from build123d import *

# Parameters (mm, degrees)
SKETCH_1_W         = 31
SKETCH_1_H         = 21
EXTRUDE_1_DEPTH    = 42
SHELL_1_T          = -1
SKETCH_2_W         = 5
SKETCH_2_H         = 21
EXTRUDE_2_DEPTH    = 6
SHELL_START        = 42
SHELL_2_OUTLINE_W  = 4
SHELL_2_OUTLINE_H  = 21
SHELL_2_DEPTH      = 6
SKETCH_3_W         = 5
SKETCH_3_H         = 21
EXTRUDE_3_DEPTH    = 6
SHELL_START_2      = -6
SHELL_3_OUTLINE_W  = 4
SHELL_3_OUTLINE_H  = 21
SHELL_3_DEPTH      = 6
SKETCH_4_W         = 21
SKETCH_4_H         = 1
EXTRUDE_4_DEPTH    = 23
SKETCH_5_W         = 21
SKETCH_5_H         = 5
EXTRUDE_5_DEPTH    = 6
SHELL_START_3      = 18
SHELL_4_OUTLINE_W  = 21
SHELL_4_OUTLINE_H  = 6
SHELL_4_DEPTH      = 4
SKETCH_6_W         = 21
SKETCH_6_H         = 5
EXTRUDE_6_DEPTH    = 6
SHELL_5_OUTLINE_W  = 21
SHELL_5_OUTLINE_H  = 6
SHELL_5_DEPTH      = 4
SKETCH_8_W         = 21
SKETCH_8_H         = 42
EXTRUDE_7_DEPTH    = 1
HOLE_WIZARD_M3_1_D = 2.5
HOLE_WIZARD_M3_2_D = 2.5
HOLE_WIZARD_M3_3_D = 2.5
HOLE_WIZARD_M3_4_D = 2.5
FILLET_2_R         = 0.5
FILLET_3_R         = 5


# Read off the part's stored shape, not the designer's step: 抽壳2, 抽壳3, 抽壳4, 抽壳5
with BuildPart() as part:
    # 草图1 → 凸台-拉伸1 (new body)
    with BuildSketch(Plane(origin=(0, 0, 0), x_dir=(1, 0, 0), z_dir=(0, 1, 0))):
        with Locations((-15.5, 10.5)):
            Rectangle(SKETCH_1_W, SKETCH_1_H)
    extrude(amount=EXTRUDE_1_DEPTH)

    # 抽壳1
    shell_1_openings = [part.faces().sort_by_distance(p)[0] for p in [
        (-15.5, 21, 0),
        (-31, 21, -10.5),
        (-15.5, 21, -21),
    ]]
    offset(amount=SHELL_1_T, openings=shell_1_openings, kind=Kind.INTERSECTION)

    # 草图2 → 凸台-拉伸2 (add)
    with BuildSketch(Plane(origin=(0, 42, 0), x_dir=(1, 0, 0), z_dir=(0, 1, 0))):
        with Locations((-28.5, 10.5)):
            Rectangle(SKETCH_2_W, SKETCH_2_H)
    extrude(amount=EXTRUDE_2_DEPTH)

    # 抽壳2 outline → 抽壳2 (cut)
    with BuildSketch(Plane(origin=(0, 0, 0), x_dir=(1, 0, 0), z_dir=(0, 1, 0)).offset(SHELL_START)):
        with Locations((-28, 10.5)):
            Rectangle(SHELL_2_OUTLINE_W, SHELL_2_OUTLINE_H)
    extrude(amount=SHELL_2_DEPTH, mode=Mode.SUBTRACT)

    # 草图3 → 凸台-拉伸3 (add)
    with BuildSketch(Plane.XZ):
        with Locations((-28.5, -10.5)):
            Rectangle(SKETCH_3_W, SKETCH_3_H)
    extrude(amount=EXTRUDE_3_DEPTH)

    # 抽壳3 outline → 抽壳3 (cut)
    with BuildSketch(Plane(origin=(0, 0, 0), x_dir=(1, 0, 0), z_dir=(0, 1, 0)).offset(SHELL_START_2)):
        with Locations((-28, 10.5)):
            Rectangle(SHELL_3_OUTLINE_W, SHELL_3_OUTLINE_H)
    extrude(amount=SHELL_3_DEPTH, mode=Mode.SUBTRACT)

    # 草图4 → 凸台-拉伸4 (add)
    with BuildSketch(Plane.XY):
        with Locations((-19.5, 41.5)):
            Rectangle(SKETCH_4_W, SKETCH_4_H)
        with Locations((-19.5, 0.5)):
            Rectangle(SKETCH_4_W, SKETCH_4_H)
    extrude(amount=EXTRUDE_4_DEPTH)

    # 草图5 → 凸台-拉伸5 (add)
    with BuildSketch(Plane(origin=(0, 42, 0), x_dir=(1, 0, 0), z_dir=(0, 1, 0))):
        with Locations((-19.5, -20.5)):
            Rectangle(SKETCH_5_W, SKETCH_5_H)
    extrude(amount=EXTRUDE_5_DEPTH)

    # 抽壳4 outline → 抽壳4 (cut)
    with BuildSketch(Plane.XY.offset(SHELL_START_3)):
        with Locations((-19.5, 45)):
            Rectangle(SHELL_4_OUTLINE_W, SHELL_4_OUTLINE_H)
    extrude(amount=SHELL_4_DEPTH, mode=Mode.SUBTRACT)

    # 草图6 → 凸台-拉伸6 (add)
    with BuildSketch(Plane.XZ):
        with Locations((-19.5, 20.5)):
            Rectangle(SKETCH_6_W, SKETCH_6_H)
    extrude(amount=EXTRUDE_6_DEPTH)

    # 抽壳5 outline → 抽壳5 (cut)
    with BuildSketch(Plane.XY.offset(SHELL_START_3)):
        with Locations((-19.5, -3)):
            Rectangle(SHELL_5_OUTLINE_W, SHELL_5_OUTLINE_H)
    extrude(amount=SHELL_5_DEPTH, mode=Mode.SUBTRACT)

    # 草图8 → 凸台-拉伸7 (add)
    with BuildSketch(Plane(origin=(0, 0, -21), x_dir=(-1, 0, 0), z_dir=(0, 0, -1))):
        with Locations((19.5, 21)):
            Rectangle(SKETCH_8_W, SKETCH_8_H)
    extrude(amount=EXTRUDE_7_DEPTH)

    # M3 螺纹孔1 (through all)
    with Locations(Plane.XY.offset(23)):
        with Locations((-24.5, 45), (-14.5, 45), (-24.5, -3), (-14.5, -3)):
            Hole(HOLE_WIZARD_M3_1_D / 2)

    # M3 螺纹孔2 (through all)
    with Locations(Plane.ZY.offset(31)):
        with Locations((-5.5, 45), (-15.5, 45), (-15.5, -3), (-5.5, -3)):
            Hole(HOLE_WIZARD_M3_2_D / 2)

    # M3 螺纹孔3 (through all)
    with Locations(Plane(origin=(0, 0, 0), x_dir=(0, 0, -1), z_dir=(1, 0, 0))):
        with Locations((10.5, 11)):
            Hole(HOLE_WIZARD_M3_3_D / 2)

    # M3 螺纹孔4 (through all)
    with Locations(Plane(origin=(0, 0, -22), x_dir=(-1, 0, 0), z_dir=(0, 0, -1))):
        with Locations((19.5, 11)):
            Hole(HOLE_WIZARD_M3_4_D / 2)

    # 圆角2
    fillet_2_edges = [part.edges().sort_by_distance(p)[0] for p in [
        (-19.5, 42, -22),
        (-19.5, 0, -22),
        (-31, 1, -10.5),
        (-31, 41, -10.5),
        (0, 42, -10.5),
        (0, 0, -10.5),
        (-19.5, 41, 23),
        (-19.5, 1, 23),
    ]]
    fillet(fillet_2_edges, radius=FILLET_2_R)

    # 圆角3
    fillet_3_edges = [part.edges().sort_by_distance(p)[0] for p in [
        (-30, 48, 22.5),
        (-9, 48, 22.5),
        (-30, -6, 22.5),
        (-9, -6, 22.5),
        (-30.5, 48, -21),
        (-30.5, 48, 0),
        (-30.5, -6, -21),
        (-30.5, -6, 0),
    ]]
    fillet(fillet_3_edges, radius=FILLET_3_R)


solid = part.part
Build history of the part. All positions in model axes, mm. A direction names the side the tool comes from. Give positions to 0.01 mm unless a question says otherwise; leave off trailing zeros. Loops run counter-clockwise (first coordinate to the right, second up) from the corner with the lowest first, then second, coordinate; pieces in that order, holes last. Notation, with made-up numbers: (-30, 71) - (-10, 71) arc R22 cw to (-10, 96) - close; hole circle Ø7 at (61.5, -23.5). An arc over 180 degrees is marked (long way). Write item = value, one per line. Start each with the question number.
1) Drop flat-ended pins along their axis: pin 1 Ø4 at (x, y) = (-12, 10) entering from +Z; pin 2 Ø1.6 at (y, z) = (0, 12.5) entering from -X; pin 3 Ø3 at (y, z) = (46, -14.5) entering from +X; pin 4 Ø2 at (x, y) = (-19.5, 11) entering from +Z. Give the stop position or say it passes through.
2) Band-saw the part on C-C on x = -17. Give the cut face in (y, z).
3) Band-saw the part on D-D on z = -13. Give the cut face in (x, y).
4) Band-saw the part on B-B on z = 12.5. Give the cut face in (x, y).
5) Band-saw the part on A-A on y = 22. Give the cut face in (x, z).
6) Pull direction Y, two halves, no side cores. Call faces 6 (the flat face through (-31, 45, -10)), 7 (the flat face through (-19, 21, -21)), 8 (the cylindrical face through (-30.49, 46.5, -19.57)): +Y half, -Y half, draft (parallel to the pull), parting line (faces both ways), or undercut.
7) Probe probe 1 along Y at (x, z) = (-30.6, -5.5); probe 2 along Y at (x, z) = (-3, -20); probe 3 along Z at (x, y) = (-26, 19). List the from-to ranges inside material, lowest first. Write a range as from..to.
8) Tool access for faces 1 (the flat face through (-30, 41.5, 11.7)), 2 (the flat face through (-18, 0, 1)), 3 (the flat face through (-16, 41, 0)), 4 (the flat face through (-30, 45, -10)), 5 (the flat face through (-0.85, 21.1, 0)): list every direction of +Z, -Z, +X, -X, +Y, -Y with a clear straight run to the whole face (end or side of a thin tool).
Final values:
q1.pin_1 = -21
q1.pin_2 = -30
q1.pin_3 = -30
q1.pin_4 = through
q2.outline = (-6, 22) - (0, 22) - (0, -21.5) arc R0.5 ccw to (0.5, -22) - (41.5, -22) arc R0.5 ccw to (42, -21.5) - (42, 22) - (48, 22) - (48, 23) - (41.5, 23) arc R0.5 ccw to (41, 22.5) - (41, -21) - (1, -21) - (1, 22.5) arc R0.5 ccw to (0.5, 23) - (-6, 23) - close
q3.outline = (-31, -6) - (-30, -6) - (-30, 0) - (-0.5, 0) arc R0.5 ccw to (0, 0.5) - (0, 41.5) arc R0.5 ccw to (-0.5, 42) - (-30, 42) - (-30, 48) - (-31, 48) - (-31, 41.5) arc R0.5 ccw to (-30.5, 41) - (-1, 41) - (-1, 1) - (-30.5, 1) arc R0.5 ccw to (-31, 0.5) - close
q4.outline = (-30, 0) - (-9, 0) - (-9, 1) - (-30, 1) - close; (-30, 41) - (-9, 41) - (-9, 42) - (-30, 42) - close
q5.outline = (-30, -22) - (-9, -22) - (-9, -21) - (-30, -21) - close; (-1, -21) - (0, -21) - (0, 0) - (-1, 0) - close
q6.face_6 = draft
q6.face_7 = undercut
q6.face_8 = +Y half
q7.probe_1 = -6..-4.25, -1.75..0.99, 41.01..43.75, 46.25..48
q7.probe_2 = 0..1, 41..42
q7.probe_3 = -22..-21
q8.face_1 = +Z, -X, +Y, -Y
q8.face_2 = -Z, +X, -Y
q8.face_3 = +Z, -X
q8.face_4 = -Z, +X, +Y
q8.face_5 = +Z, +X, +Y, -Y
